Answer from the drawing. Dimensions are ordinates in mm from the lowest x, y and z of the part. A direction names the side the tool comes from. Coordinates: 2 decimals unless noted, no trailing zeros. Write each loop counter-clockwise with the first axis right and the second up, starting at its lowest first coordinate (ties: lowest second). Pieces come first, ordered by that corner, then holes. Notation, with made-up numbers: (-36, -38.75) - (-2, -38.75) arc R6 cw to (-2, -32.75) - close; hole circle Ø11 at (38.5, 17.25). An arc over 180 degrees is marked (long way). Use one line per item in the form item = value. Start each with the question number.
Item 1: Consider probe 1 along Z at (x, y) = (5.5, 11.5); probe 2 along Y at (x, z) = (25.5, 16.5); probe 3 along X at (y, z) = (29, 19). Determine where each line is inside the solid, lowest interval first.
Item 2: Given pin 1 (11 mm diameter, centred on x = 20, z = 36, fed in from +Y); pin 2 (6 mm diameter, centred on x = 29.5, z = 13.5, fed in from -Y); pin 3 (12 mm diameter, centred on y = 31, z = 10.5, fed in from +X), each flat-ended and moving along its own axis, determine where each tip first touches the part or whether it passes through.
Item 3: A cutting plane is placed at D-D (y = 57). Write down the section's boundary in (x, z).
Item 4: A cutting plane is placed at B-B (x = 20). Write down the section's boundary in (y, z).
Item 5: A cutting plane is placed at A-A (y = 17.5). Write down the section's boundary in (x, z).
Item 6: For the marked faces 1, 2 and 3, determine the directions among +Z, -Z, +X, -X, +Y, -Y from which every point of the face is accessible in a straight line to the end or side of a thin tool.
Item 7: A cutting plane is placed at C-C (z = 13.5). Write down the section's boundary in (x, y), then the cut area to 3 significant figures.
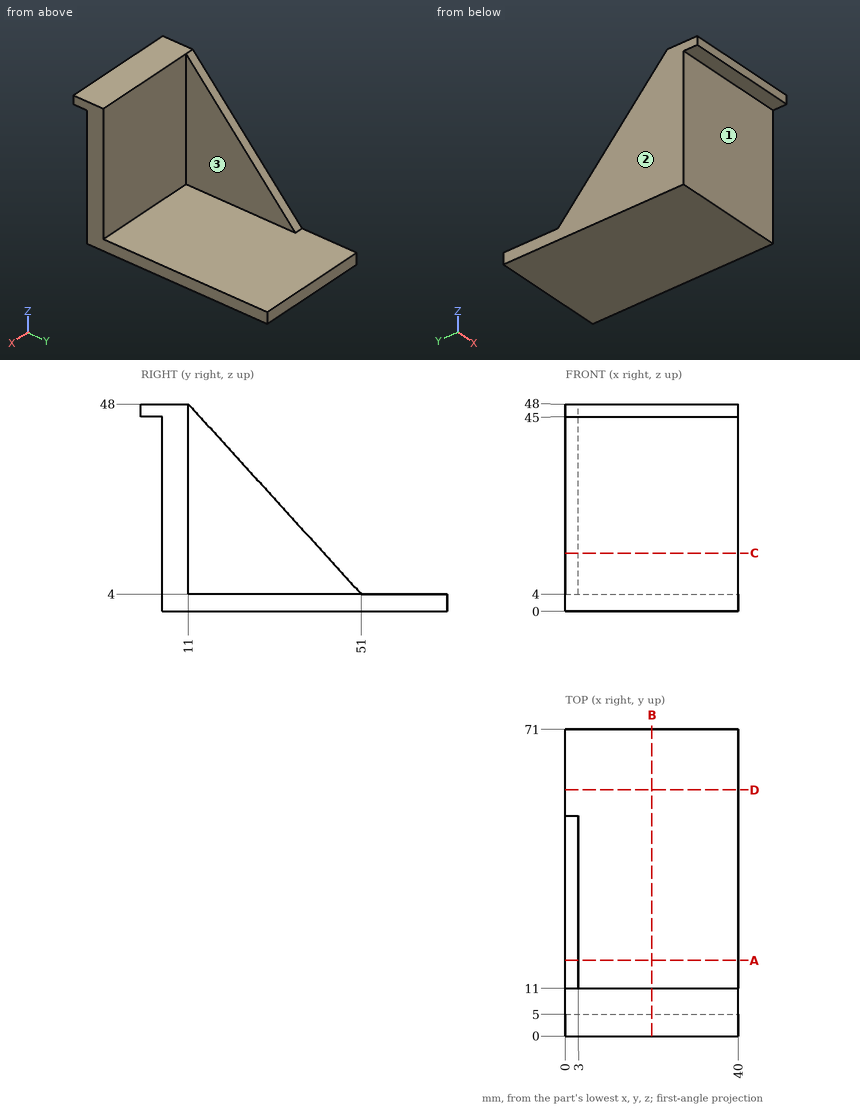
Answer:
q1.probe_1 = 0 to 4
q1.probe_2 = 5 to 11
q1.probe_3 = 0 to 3
q2.pin_1 = 11
q2.pin_2 = 5
q2.pin_3 = 3
q3.outline = (0, 0) - (40, 0) - (40, 4) - (0, 4) - close
q4.outline = (0, 45) - (5, 45) - (5, 0) - (71, 0) - (71, 4) - (11, 4) - (11, 48) - (0, 48) - close
q5.outline = (0, 0) - (40, 0) - (40, 4) - (3, 4) - (3, 40.85) - (0, 40.85) - close
q6.face_1 = -Z, +X, -X, -Y
q6.face_2 = +Z, -Z, -X, +Y, -Y
q6.face_3 = +Z, +X, +Y
q7.outline = (0, 5) - (40, 5) - (40, 11) - (3, 11) - (3, 42.36) - (0, 42.36) - close
q7.area = 334 mm²
